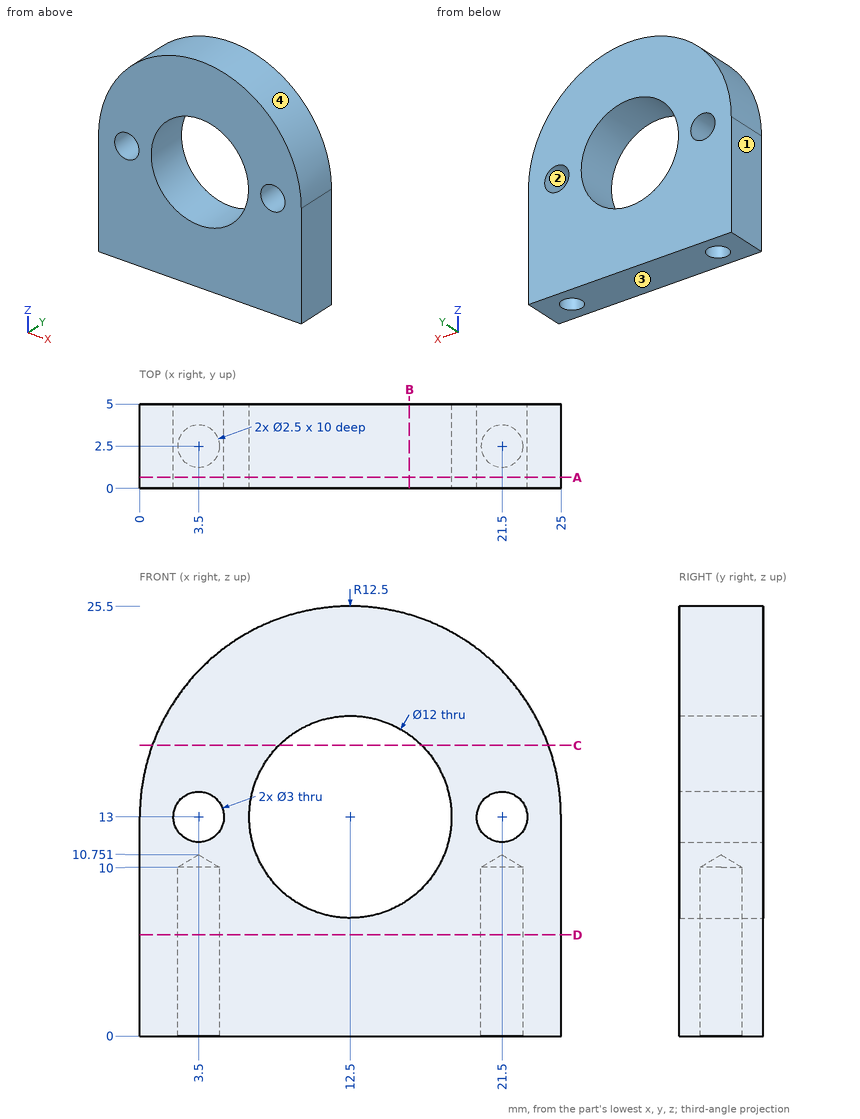
Study the drawing (mm; zero at the part's minimum x, y, z) and answer. Round coordinates to 2 decimals unless told otherwise and drop trailing zeros. Write each loop counter-clockwise with the first axis right and the second up, starting at its lowest first coordinate (ties: lowest second). Pieces come first, ordered by that corner, then holes.
1) A cutting plane is placed at A-A (y = 0.65). Give the vertices of the cut face in (x, z).
2) The mould has two halves that part along X. Classify the marked faces 1, 2, 3 and 4: pulls with the +X half, pulls with the -X half, needs draft (parallel to the pull), parting line crosses it, or undercut.
3) A cutting plane is placed at B-B (x = 16). Give the vertices of the cut face in (y, z), plus the area to 3 significant figures.
4) A cutting plane is placed at C-C (z = 17.25). Give the vertices of the cut face in (x, y).
5) Straight lines are drawn through the part: line 1 (X direction, y = 1.65, z = 13); line 2 (X direction, y = 2.5, z = 5); line 3 (Y direction, x = 3.5, z = 3.5). For each, find the intervals that lie inside material, in ascending order.
6) A cutting plane is placed at D-D (z = 6). Give the vertices of the cut face in (x, y).
7) Given pin 1 Ø1 at (x, y) = (19, 2) entering from +Z; pin 2 Ø1 at (x, y) = (17.5, 3) entering from -Z; pin 3 Ø2 at (x, y) = (21.5, 2.5) entering from -Z, each flat-ended and moving along its own axis, determine where each tip first touches the part or whether it passes through.
Completed:
1. outline: (0, 0) - (25, 0) - (25, 13) arc R12.5 ccw to (0, 13) - close; hole circle Ø3 at (3.5, 13); hole circle Ø12 at (12.5, 13); hole circle Ø3 at (21.5, 13)
2. face 1: pulls with the -X half
2. face 2: undercut
2. face 3: needs draft
2. face 4: parting line crosses it
3. outline: (0, 0) - (5, 0) - (5, 8.13) - (0, 8.13) - close; (0, 17.87) - (5, 17.87) - (5, 25) - (0, 25) - close
3. area: 76.3 mm2
4. outline: (0.74, 0) - (8.26, 0) - (8.26, 5) - (0.74, 5) - close; (16.74, 0) - (24.26, 0) - (24.26, 5) - (16.74, 5) - close
5. line 1: x = 0 to 2, 5 to 6.5, 18.5 to 20, 23 to 25
5. line 2: x = 0 to 2.25, 4.75 to 20.25, 22.75 to 25
5. line 3: y = 0 to 1.25, 3.75 to 5
6. outline: (0, 0) - (25, 0) - (25, 5) - (0, 5) - close; hole circle Ø2.5 at (3.5, 2.5); hole circle Ø2.5 at (21.5, 2.5)
7. pin 1: stops at z = 23.97
7. pin 2: stops at z = 0
7. pin 3: stops at z = 10.15
